from build123d import *

# Parameters (mm, degrees)
SKETCH1_W           = 77
SKETCH1_H           = 77
BOSS_EXTRUDE1_DEPTH = 5
SKETCH2_W           = 87
SKETCH2_H           = 87
SKETCH2_W_2         = 77
SKETCH2_H_2         = 77
BOSS_EXTRUDE2_DEPTH = 33
SKETCH3_R           = 3.5
SKETCH3_R_2         = 2
BOSS_EXTRUDE4_DEPTH = 18.5
SKETCH11_W          = 1.5
SKETCH11_H          = 28
BOSS_EXTRUDE7_DEPTH = 1.5
BOSS_EXTRUDE8_DEPTH = 4
SKETCH7_R           = 4
CUT_EXTRUDE1_DEPTH  = 2
CUT_EXTRUDE2_DEPTH  = 5
SKETCH16_W          = 10
SKETCH16_H          = 5
CUT_EXTRUDE3_DEPTH  = 5
BOSS_EXTRUDE6_DEPTH = 7.5
FILLET1_R           = 2
FILLET2_R           = 1
CHAMFER1_SIZE       = 3


with BuildPart() as part:
    # Sketch1 → Boss-Extrude1 (new body)
    with BuildSketch(Plane(origin=(0, 0, 0), x_dir=(1, 0, 0), z_dir=(0, 1, 0))):
        Rectangle(SKETCH1_W, SKETCH1_H)
    extrude(amount=BOSS_EXTRUDE1_DEPTH)

    # Sketch2 → Boss-Extrude2 (add)
    with BuildSketch(Plane(origin=(0, 0, 0), x_dir=(1, 0, 0), z_dir=(0, 1, 0))):
        Rectangle(SKETCH2_W, SKETCH2_H)
        Rectangle(SKETCH2_W_2, SKETCH2_H_2, mode=Mode.SUBTRACT)
    extrude(amount=BOSS_EXTRUDE2_DEPTH)

    # Sketch3 → Boss-Extrude4 (add)
    # profile 1 of 4: a face of its own
    with BuildSketch(Plane(origin=(0, 5, 0), x_dir=(1, 0, 0), z_dir=(0, 1, 0))):
        with Locations(Location((-28.5, -19, 0), (0, 0, 90))):
            Circle(SKETCH3_R)
        with Locations(Location((-28.5, -19, 0), (0, 0, 270))):
            Circle(SKETCH3_R_2, mode=Mode.SUBTRACT)
    # profile 2 of 4: a face of its own
    with BuildSketch(Plane(origin=(0, 5, 0), x_dir=(1, 0, 0), z_dir=(0, 1, 0))):
        with Locations(Location((-19, 19, 0), (0, 0, 90))):
            Circle(SKETCH3_R)
        with Locations(Location((-19, 19, 0), (0, 0, 270))):
            Circle(SKETCH3_R_2, mode=Mode.SUBTRACT)
    # profile 3 of 4: a face of its own
    with BuildSketch(Plane(origin=(0, 5, 0), x_dir=(1, 0, 0), z_dir=(0, 1, 0))):
        with Locations(Location((28.5, -19, 0), (0, 0, 90))):
            Circle(SKETCH3_R)
        with Locations(Location((28.5, -19, 0), (0, 0, 270))):
            Circle(SKETCH3_R_2, mode=Mode.SUBTRACT)
    # profile 4 of 4: a face of its own
    with BuildSketch(Plane(origin=(0, 5, 0), x_dir=(1, 0, 0), z_dir=(0, 1, 0))):
        with Locations(Location((19, 19, 0), (0, 0, 90))):
            Circle(SKETCH3_R)
        with Locations(Location((19, 19, 0), (0, 0, 270))):
            Circle(SKETCH3_R_2, mode=Mode.SUBTRACT)
    extrude(amount=BOSS_EXTRUDE4_DEPTH)

    # Sketch11 → Boss-Extrude7 (add)
    with BuildSketch(Plane(origin=(0, 5, 0), x_dir=(1, 0, 0), z_dir=(0, 1, 0))):
        with Locations((4.75, 24.5)):
            Rectangle(SKETCH11_W, SKETCH11_H)
        with Locations((-4.75, 24.5)):
            Rectangle(SKETCH11_W, SKETCH11_H)
    extrude(amount=BOSS_EXTRUDE7_DEPTH)

    # Sketch17 → Boss-Extrude8 (add)
    with BuildSketch(Plane(origin=(0, 5, 0), x_dir=(1, 0, 0), z_dir=(0, 1, 0))):
        Polygon((-8.89, 10.5), (-8.89, 5.5), (8.89, 5.5), (8.89, 10.5), (11.89, 10.5), (11.89, 3), (-11.89, 3), (-11.89, 10.5), align=None)
    extrude(amount=BOSS_EXTRUDE8_DEPTH)

    # Sketch7 → Cut-Extrude1 (cut)
    with BuildSketch(Plane.XZ):
        with Locations(Location((-23.5, -23.5, 0), (0, 0, 270))):
            Circle(SKETCH7_R)
        with Locations(Location((-23.5, 23.5, 0), (0, 0, 270))):
            Circle(SKETCH7_R)
        with Locations(Location((23.5, 23.5, 0), (0, 0, 270))):
            Circle(SKETCH7_R)
        with Locations(Location((23.5, -23.5, 0), (0, 0, 270))):
            Circle(SKETCH7_R)
    extrude(amount=-CUT_EXTRUDE1_DEPTH, mode=Mode.SUBTRACT)

    # Sketch10 → Cut-Extrude2 (cut)
    with BuildSketch(Plane(origin=(0, 0, -38.5), x_dir=(-1, 0, 0), z_dir=(0, 0, -1))):
        with BuildLine():
            Line((-5, 13), (5, 13))
            ThreePointArc((5, 13), (7.5, 10.5), (5, 8))
            Line((5, 8), (-5, 8))
            ThreePointArc((-5, 8), (-7.5, 10.5), (-5, 13))
        make_face()
    extrude(amount=CUT_EXTRUDE2_DEPTH, mode=Mode.SUBTRACT)

    # Sketch16 → Cut-Extrude3 (cut)
    with BuildSketch(Plane.ZY.offset(-38.5)):
        with Locations((-23.5, 7.5)):
            Rectangle(SKETCH16_W, SKETCH16_H)
    extrude(amount=-CUT_EXTRUDE3_DEPTH, mode=Mode.SUBTRACT)

    # Sketch15 → Boss-Extrude6 (add)
    with BuildSketch(Plane(origin=(0, 5, 0), x_dir=(1, 0, 0), z_dir=(0, 1, 0))):
        Polygon((-11, -0.5), (-11, -8.5), (-13, -8.5), (-13, 1.5), (-6, 1.5), (-6, -0.5), align=None)
        Polygon((-13, -24.5), (-11, -24.5), (-11, -32.5), (-6, -32.5), (-6, -34.5), (-13, -34.5), align=None)
        Polygon((13, -24.5), (11, -24.5), (11, -32.5), (6, -32.5), (6, -34.5), (13, -34.5), align=None)
        Polygon((6, 1.5), (6, -0.5), (11, -0.5), (11, -8.5), (13, -8.5), (13, 1.5), align=None)
    extrude(amount=BOSS_EXTRUDE6_DEPTH)

    # Fillet1
    fillet1_edges = [part.edges().sort_by_distance(p)[0] for p in [
        (28.5, 5, 22.5),
        (19, 5, -15.5),
        (-28.5, 5, 22.5),
        (-19, 5, -15.5),
    ]]
    fillet(fillet1_edges, radius=FILLET1_R)

    # Fillet2
    fillet2_edges = [part.edges().sort_by_distance(p)[0] for p in [
        (-8.89, 7, -10.5),
        (-11.89, 7, -10.5),
        (-11.89, 7, -3),
        (11.89, 7, -3),
        (11.89, 7, -10.5),
        (8.89, 7, -10.5),
        (-13, 8.75, -1.5),
        (13, 8.75, -1.5),
        (-13, 8.75, 34.5),
        (13, 8.75, 34.5),
    ]]
    fillet(fillet2_edges, radius=FILLET2_R)

    # Chamfer1
    chamfer1_edges = [part.edges().sort_by_distance(p)[0] for p in [
        (-43.5, 16.5, 43.5),
        (43.5, 16.5, 43.5),
        (43.5, 16.5, -43.5),
        (-43.5, 16.5, -43.5),
    ]]
    chamfer(chamfer1_edges, length=CHAMFER1_SIZE)


solid = part.part
CAD build for the part. Positions are in the model's coordinates, mm. A direction names the side the tool comes from. Round coordinates to 2 decimals unless told otherwise and drop trailing zeros.
(1) Drop flat-ended pins along their axis: P1, Ø4.5, axis at x = -29, z = 18, coming from the +Y side; P2, Ø1, axis at x = -2.5, z = -29, coming from the +Y side; P3, Ø7, axis at x = 23.5, z = 23.5, coming from the -Y side. Give the stop position or say it passes through.
(2) 3-axis set-ups, long thin cutter, end or side, ignore diameter. For faces 5 (the face through (41, 7, -18.5)), 6 (the face through (-1, 19, -38.5)): which of +Z, -Z, +X, -X, +Y, -Y reach the whole face in a straight line?
(3) Probe line 1 along X through (y, z) = (19.5, 19); line 2 along Z through (x, y) = (16, 28.5); line 3 along Z through (x, y) = (9.5, 7.5). List the from-to ranges inside material, lowest first.
(4) Mould opens along Z. For faces 1 (the face through (8.89, 7, -7)), 2 (the face through (43.5, 16, 1)), 3 (the face through (-6, 9, -1)), 4 (the face through (-1, 16, 43.5)) say: pulls with the +Z half, pulls with the -Z half, needs draft (parallel to the pull), parting line crosses it, or undercut.
From the geometry:
1. P1: stops at y = 23.5
1. P2: stops at y = 5
1. P3: stops at y = 2
2. face 5: +X
2. face 6: +Y
3. line 1: x = -43.5 to -38.5, -32 to -30.5, -26.5 to -25, 25 to 26.5, 30.5 to 32, 38.5 to 43.5
3. line 2: z = -43.5 to -38.5, 38.5 to 43.5
3. line 3: z = -43.5 to -38.5, -10.42 to -3, -1.5 to 0.5, 32.5 to 34.5, 38.5 to 43.5
4. face 1: undercut
4. face 2: needs draft
4. face 3: undercut
4. face 4: pulls with the +Z half
